Source: three-view drawing plus pictorial views. Frame: mm from the lowest corner of the part. A direction names the side the tool comes from. Round coordinates to 2 decimals unless told otherwise and drop trailing zeros. Loops run counter-clockwise (first coordinate to the right, second up) from the corner with the lowest first, then second, coordinate; pieces in that order, holes last. Notation, with made-up numbers: M 84,55 L 136,55 A21 ccw 136,77 Z; hole C -15,11 d6. An arc over 180 degrees is marked long. Return JSON: item names as keys, results as strings. Group by question number.
1) Access query for the marked faces 1, 2 and 3. Directions: +Z, -Z, +X, -X, +Y, -Y. A direction counts if a zero-diameter tool reaches every point of the face in a straight line with its end or side. Return the directions, or none.
2) Section A-A (y = 7.75). Output: boundary loops of the cut face in (x, z) (1 decimal), plus the area to 3 significant figures.
3) Section C-C (x = 5). Output: boundary loops of the cut face in (y, z).
4) Material intervals for line 1 (X direction, y = 9.75, z = 11.75) (1 decimal); line 2 (Z direction, x = 2, y = 8.5) (1 decimal); line 3 (Z direction, x = 19.5, y = 8.5), sorted ascending. Write a range as from..to.
5) Section B-B (z = 19). Output: boundary loops of the cut face in (x, y) (1 decimal), plus the area to 3 significant figures.
6) Contact query for flat-ended pins moving along their axis: P1, Ø2, axis at x = 14.5, z = 5.5, coming from the -Y side; P2, Ø1.5, axis at x = 18, y = 7.5, coming from the -Z side; P3, Ø4, axis at x = 6, y = 1.5, coming from the -Z side; P4, Ø3.5, axis at x = 3.5, y = 2.5, coming from the +Z side. Output: stop coordinate, or through.
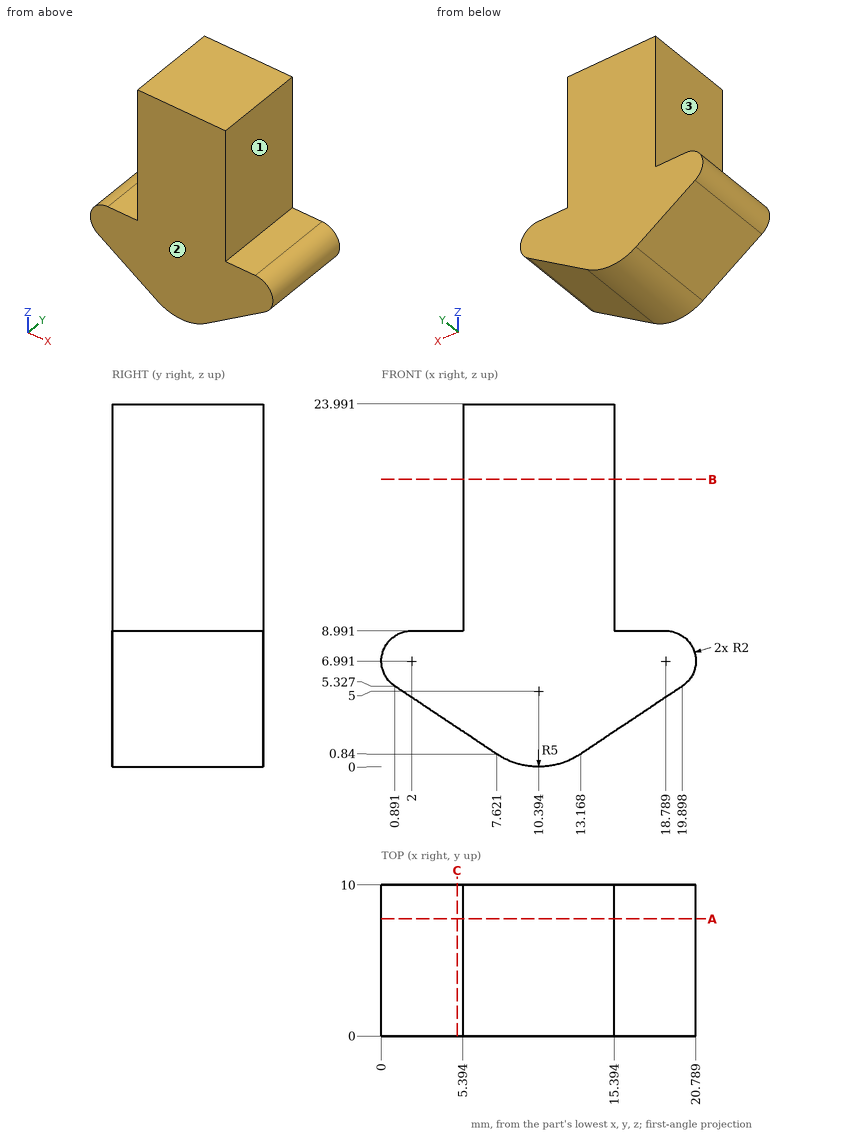
Returned:
{
 "1": {"face 1": "+Z, +X, +Y, -Y", "face 2": "+Z, -Z, +X, -X, -Y", "face 3": "+Z, -X, +Y, -Y"},
 "2": {"outline": "M 0.9,5.3 L 7.6,0.8 A5 ccw 13.2,0.8 L 19.9,5.3 A2 ccw 18.8,9 L 15.4,9 L 15.4,24 L 5.4,24 L 5.4,9 L 2,9 A2 ccw Z", "area": "282 mm^2"},
 "3": {"outline": "M 0,2.59 L 10,2.59 L 10,8.99 L 0,8.99 Z"},
 "4": {"line 1": "x = 5.4..15.4", "line 2": "z = 4.6..9", "line 3": "z = 5.06..8.86"},
 "5": {"outline": "M 5.4,0 L 15.4,0 L 15.4,10 L 5.4,10 Z", "area": "100 mm^2"},
 "6": {"P1": "stops at y = 0", "P2": "stops at z = 3.56", "P3": "stops at z = 0.61", "P4": "stops at z = 8.99"}
}
